Here's how the part is built. I have some questions about the finished solid (model axes, mm). Give positions to 0.01 mm unless a question says otherwise; leave off trailing zeros. Write each loop counter-clockwise with the first axis right and the second up, starting at its lowest first coordinate (ties: lowest second). Pieces come first, ordered by that corner, then holes. Notation, with made-up numbers: M 28,37 L 45,37 A10 ccw 45,50 Z; hole C 24.25,88.5 d4. An arc over 180 degrees is marked long. Use one line per item in the form item = value. Start each with the question number.
from build123d import *

# Parameters (mm, degrees)
SZKIC1_W                    = 16
SZKIC1_H                    = 31.855734842
DODANIE_WYCI_GNI_CIE1_DEPTH = 2
SZKIC2_W                    = 16
SZKIC2_H                    = 5
WYTNIJ_WYCI_GNI_CIE1_DEPTH  = 5
WYTNIJ_WYCI_GNI_CIE2_DEPTH  = 10
WYTNIJ_WYCI_GNI_CIE3_DEPTH  = 10


with BuildPart() as part:
    # Szkic1 → Dodanie-wyciągnięcie1 (new body)
    with BuildSketch(Plane.XY):
        with Locations((8, 15.927867421)):
            Rectangle(SZKIC1_W, SZKIC1_H)
    extrude(amount=DODANIE_WYCI_GNI_CIE1_DEPTH)

    # Szkic2 → Wytnij-wyciągnięcie1 (cut)
    with BuildSketch(Plane.XY.offset(2)):
        with Locations((8, 2.5)):
            Rectangle(SZKIC2_W, SZKIC2_H)
    extrude(amount=-WYTNIJ_WYCI_GNI_CIE1_DEPTH, mode=Mode.SUBTRACT)

    # Szkic6 → Wytnij-wyciągnięcie2 (cut)
    with BuildSketch(Plane(origin=(0, 0, 0), x_dir=(-1, 0, 0), z_dir=(0, 0, -1))):
        with BuildLine():
            Line((0, 31.855734842), (-16, 31.855734842))
            Line((-16, 31.855734842), (-16, 18.750886073))
            ThreePointArc((-16, 18.750886073), (-8.06030582, 15.602264045), (0, 18.427867421))
            Line((0, 18.427867421), (0, 31.855734842))
        make_face()
    extrude(amount=-WYTNIJ_WYCI_GNI_CIE2_DEPTH, mode=Mode.SUBTRACT)

    # Szkic8 → Wytnij-wyciągnięcie3 (cut)
    with BuildSketch(Plane(origin=(0, 0, 0), x_dir=(-1, 0, 0), z_dir=(0, 0, -1))):
        with BuildLine():
            Line((-16, 18.750886073), (-16, 16.446330699))
            ThreePointArc((-16, 16.446330699), (-8.074613492, 13.210416858), (0, 16.05356769))
            Line((0, 16.05356769), (0, 18.427867421))
            Line((0, 18.427867421), (-16, 18.750886073))
        make_face()
    extrude(amount=-WYTNIJ_WYCI_GNI_CIE3_DEPTH, mode=Mode.SUBTRACT)


solid = part.part
1) Suppose I cut it at C-C, the plane x = 13.75. List the corners of the cut face in (y, z) for me, and give its area (3 significant figures).
2) Suppose I cut it at B-B, the plane z = 0.9. List the corners of the cut face in (x, y) for me.
3) Will this pin go through, and if not, where does the flat tip stop? P1, Ø3, axis at x = 6.5, y = 13, coming from the -Z side.
4) Suppose I cut it at A-A, the plane y = 15. List the corners of the cut face in (x, z) for me, and give its area (3 significant figures).
5) Please list where these lines run through material, in increasing order: line 1 (Y direction, x = 11.5, z = 1); line 2 (Y direction, x = 1.75, z = 0.65).
6) Thinking about a two-plate mould opening in X: for faces 1 (the face through (16, 11, 1)), 2 (the face through (8.197, 13.214, 0.986)), 3 (the face through (8, 10, 0)), which applies, released by +X, released by -X, zero draft, split by the parting line, or undercut?
Checks:
q1.outline = M 5,0 L 14.79,0 L 14.79,2 L 5,2 Z
q1.area = 19.6 mm^2
q2.outline = M 0,5 L 16,5 L 16,16.45 A12.05 cw 0,16.05 Z
q3.P1 = 0
q4.outline = M 0,0 L 1.45,0 L 1.45,2 L 0,2 Z; M 14.1,0 L 16,0 L 16,2 L 14.1,2 Z
q4.area = 6.70 mm^2
q5.line_1 = 5 to 13.8
q5.line_2 = 5 to 14.82
q6.face_1 = released by +X
q6.face_2 = undercut
q6.face_3 = zero draft
